Geometry: final body of the model. Coordinates: model frame, mm. Face numbers are marked on the shaded views. A direction names the side the tool comes from. Coordinates: 2 decimals unless noted, no trailing zeros. Order: outer loops, then holes, each group sorted by start corner. A loop starts at its lowest first (then second) coordinate and runs counter-clockwise, first axis right, second up. Notation, with made-up numbers: (88.25, 27) - (130.25, 27) arc R23 ccw to (130.25, 47) - close; hole circle Ø3 at (22.25, 85.5). An arc over 180 degrees is marked (long way). Use a Markdown table: item, result. Add a question column.
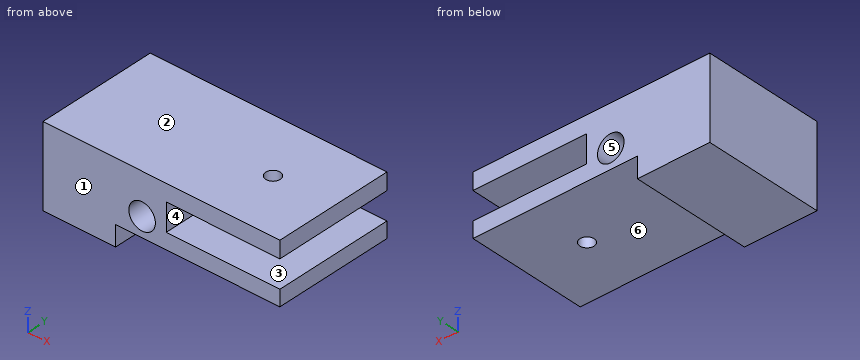
```python
from build123d import *

# Parameters (mm, degrees)
F0_W      = 366
F0_H      = 33.5
F1_DEPTH  = 25
F2_W      = 50
F2_H      = 11.4
F3_DEPTH  = 47
F4_W      = 50
F4_H      = 11.4
F5_DEPTH  = 53
F6_W      = 68
F6_H      = 8.5
F7_DEPTH  = 100
F8_W      = 170
F8_H      = 21
F9_DEPTH  = 79.8
F10_R     = 11.5
F11_DEPTH = 56
F12_W     = 78.038405627
F12_H     = 72.1084345132
F13_DEPTH = 268.001
F14_R     = 3
F15_DEPTH = 50
F16_R     = 5.5
F17_DEPTH = 100


with BuildPart() as f1:
    # F0 (on Front) → F1 (new body, symmetric)
    with BuildSketch(Plane.XZ):
        with Locations((0, 16.75)):
            Rectangle(F0_W, F0_H)
    extrude(amount=F1_DEPTH, both=True)

    # F2 (on face) → F3 (cut)
    with BuildSketch(Plane.YZ.offset(183)):
        with Locations((0, 20.8)):
            Rectangle(F2_W, F2_H)
    extrude(amount=-F3_DEPTH, mode=Mode.SUBTRACT)

    # F4 (on face) → F5 (cut)
    with BuildSketch(Plane(origin=(-183, 0, 0), x_dir=(0, -1, 0), z_dir=(-1, 0, 0))):
        with Locations((0, 20.8)):
            Rectangle(F4_W, F4_H)
    extrude(amount=-F5_DEPTH, mode=Mode.SUBTRACT)

    # F6 (on face) → F7 (cut)
    with BuildSketch(Plane.XZ.offset(25)):
        with Locations((-149, 4.25)):
            Rectangle(F6_W, F6_H)
        with Locations((149, 4.25)):
            Rectangle(F6_W, F6_H)
    extrude(amount=-F7_DEPTH, mode=Mode.SUBTRACT)

    # F8 (on face) → F9 (cut)
    with BuildSketch(Plane.XZ.offset(25)):
        with Locations((0, 23)):
            Rectangle(F8_W, F8_H)
    extrude(amount=-F9_DEPTH, mode=Mode.SUBTRACT)

    # F10 (on face) → F11 (cut)
    with BuildSketch(Plane.XY.offset(12.5)):
        Circle(F10_R)
    extrude(amount=-F11_DEPTH, mode=Mode.SUBTRACT)

    # F12 (on face) → F13 (cut, through all)
    with BuildSketch(Plane(origin=(85, 0, 0), x_dir=(0, -1, 0), z_dir=(-1, 0, 0))):
        with Locations((0.1186002046, 15.0473779067)):
            Rectangle(F12_W, F12_H)
    extrude(amount=F13_DEPTH, mode=Mode.SUBTRACT)

    # F14 (on face) → F15 (cut)
    with BuildSketch(Plane.XY.offset(33.5)):
        with Locations((158, 0)):
            Circle(F14_R)
    extrude(amount=-F15_DEPTH, mode=Mode.SUBTRACT)

    # F16 (on face) → F17 (cut)
    with BuildSketch(Plane.XZ.offset(25)):
        with Locations((126, 16.5)):
            Circle(F16_R)
    extrude(amount=-F17_DEPTH, mode=Mode.SUBTRACT)


solid = f1.part
```
1) Set-up query: the marked faces 4, 5 and 6. Return all of +Z, -Z, +X, -X, +Y, -Y with unobstructed straight access to the full face (end or side cutting, diameter ignored); none if empty.
2) Ray query, line 1 along Y through (x, z) = (158, 30); line 2 along Z through (x, y) = (150, -8); line 3 along Z through (x, y) = (126, 4). Return the intervals inside material, ascending.
3) Section C-C (x = 176). Return loops of the section in (y, z), then the cut area to 3 significant figures.
4) Draft query along Z for the marked faces 1, 2 and 3. Return one class per face: pulls with the +Z half, pulls with the -Z half, needs draft (parallel to the pull), parting line crosses it, or undercut.
5) Section D-D (z = 16.5). Return loops of the section in (x, y).
6) Section A-A (x = 158). Return loops of the section in (y, z).
7) Section B-B (y = -21). Return loops of the section in (x, z), then the cut area to 3 significant figures.
8) Pin query (flat end, axial travel): pin 1 (23.5 mm diameter, centred on x = 158, y = -4.5, fed in from -Z); pin 2 (5.5 mm diameter, centred on x = 158, y = 0, fed in from -Z); pin 3 (3.5 mm diameter, centred on y = 11, z = 20, fed in from +X); pin 4 (7 mm diameter, centred on y = 8, z = 4.5, fed in from +X). Return the tip coordinate at first contact, or that it passes through.
Values follow:
| question | item | result |
|---|---|---|
| 1 | face 4 | +X, +Y, -Y |
| 1 | face 5 | +Y, -Y |
| 1 | face 6 | -Z, +X, +Y, -Y |
| 2 | line 1 | y = -25 to -3, 3 to 25 |
| 2 | line 2 | z = 8.5 to 15.1, 26.5 to 33.5 |
| 2 | line 3 | z = 8.5 to 11, 22 to 33.5 |
| 3 | outline | (-25, 8.5) - (25, 8.5) - (25, 15.1) - (-25, 15.1) - close; (-25, 26.5) - (25, 26.5) - (25, 33.5) - (-25, 33.5) - close |
| 3 | area | 680 mm² |
| 4 | face 1 | needs draft |
| 4 | face 2 | pulls with the +Z half |
| 4 | face 3 | undercut |
| 5 | outline | (85, -25) - (120.5, -25) - (120.5, 25) - (85, 25) - close; (131.5, -25) - (136, -25) - (136, 25) - (131.5, 25) - close |
| 6 | outline | (-25, 8.5) - (-3, 8.5) - (-3, 15.1) - (-25, 15.1) - close; (-25, 26.5) - (-3, 26.5) - (-3, 33.5) - (-25, 33.5) - close; (3, 8.5) - (25, 8.5) - (25, 15.1) - (3, 15.1) - close; (3, 26.5) - (25, 26.5) - (25, 33.5) - (3, 33.5) - close |
| 7 | outline | (85, 0) - (115, 0) - (115, 8.5) - (183, 8.5) - (183, 15.1) - (136, 15.1) - (136, 26.5) - (183, 26.5) - (183, 33.5) - (85, 33.5) - close; hole circle Ø11 at (126, 16.5) |
| 7 | area | 2,070 mm² |
| 8 | pin 1 | stops at z = 8.5 |
| 8 | pin 2 | passes through |
| 8 | pin 3 | stops at x = 136 |
| 8 | pin 4 | stops at x = 115 |
